Input: part model. Units: mm. Frame: model coordinates. A direction names the side the tool comes from. Give positions to 0.01 mm unless a question says otherwise; leave off trailing zeros. Order: outer loops, then holes, each group sorted by start corner. A loop starts at its lowest first (then second) coordinate and runs counter-clockwise, first axis right, second up. Notation, with made-up numbers: M 16,-31.75 L 42,-31.75 A35 ccw 42,0.25 Z; hole C 77,-28 d1. An arc over 180 degrees is marked long. Use a Markdown table: item, result.
from build123d import *

# Parameters (mm, degrees)
SKETCH1_W           = 76.2
SKETCH1_H           = 25.4
SKETCH1_W_2         = 70.104
SKETCH1_H_2         = 19.304
BOSS_EXTRUDE1_DEPTH = 241.091915
SKETCH3_W           = 76.2
SKETCH3_H           = 25.4
SKETCH3_W_2         = 70.104
SKETCH3_H_2         = 19.304
BOSS_EXTRUDE2_DEPTH = 3.048
CUT_EXTRUDE2_START  = 104.493944
SKETCH5_R           = 38.1
CUT_EXTRUDE2_DEPTH  = 115.162609


with BuildPart() as part:
    # Sketch1 → Boss-Extrude1 (new body)
    with BuildSketch(Plane(origin=(0, 0, 0), x_dir=(1, 0, 0), z_dir=(0, 1, 0))):
        Rectangle(SKETCH1_W, SKETCH1_H)
        Rectangle(SKETCH1_W_2, SKETCH1_H_2, mode=Mode.SUBTRACT)
    extrude(amount=BOSS_EXTRUDE1_DEPTH)

    # Sketch3 → Boss-Extrude2 (add)
    with BuildSketch(Plane(origin=(0, 241.09191526, 0), x_dir=(1, 0, 0), z_dir=(0, 1, 0))):
        Rectangle(SKETCH3_W, SKETCH3_H)
        Rectangle(SKETCH3_W_2, SKETCH3_H_2, mode=Mode.SUBTRACT)
    extrude(amount=BOSS_EXTRUDE2_DEPTH)

    # Sketch5 → Cut-Extrude2 (cut)
    with BuildSketch(Plane(origin=(-101.44355263, 327.150922863, -35.760832037), x_dir=(0.275534909, -0.073492792, -0.958477607), z_dir=(0.736418318, -0.624735905, 0.259601829)).offset(CUT_EXTRUDE2_START)):
        Circle(SKETCH5_R)
    extrude(amount=CUT_EXTRUDE2_DEPTH, mode=Mode.SUBTRACT)


solid = part.part
1) Cut plane A-A on y = 83.5. Return loops of the section in (x, z).
Response values:
| item | result |
|---|---|
| outline | M -38.1,-12.7 L 38.1,-12.7 L 38.1,12.7 L -38.1,12.7 Z; hole M -35.05,-9.65 L 35.05,-9.65 L 35.05,9.65 L -35.05,9.65 Z |
2) Reachability of faces 1 (the face through (-35.052, 110, 0)), 2 (the face through (-3, 0, 10)) from +Z, -Z, +X, -X, +Y, -Y: full face, straight path, thin tool, end or side. Return the list, or none.
Response values:
| item | result |
|---|---|
| face 1 | +Y, -Y |
| face 2 | +Z, -Z, +X, -X, -Y |
3) First-contact query: pin 1 Ø12 at (y, z) = (187.5, 4.5) entering from +X. Flat tip, straight axial feed; report the tip coordinate or a pass-through.
Response values:
| item | result |
|---|---|
| pin 1 | stops at x = 7.97 |
4) Material intervals for line 1 (Z direction, x = 8, y = 10); line 2 (X direction, y = 12, z = 8.25); line 3 (X direction, y = 198.5, z = 8), sorted ascending. Write a range as from..to.
Response values:
| item | result |
|---|---|
| line 1 | z = -12.7..-9.65, 9.65..12.7 |
| line 2 | x = -38.1..-35.05, 35.05..38.1 |
| line 3 | x = -38.1..-35.05 |
